Check sheet for the modelled part. Datum: model origin and axes. Units: mm. A direction names the side the tool comes from. Round coordinates to 2 decimals unless told otherwise and drop trailing zeros. Loops run counter-clockwise (first coordinate to the right, second up) from the corner with the lowest first, then second, coordinate; pieces in that order, holes last. Notation, with made-up numbers: (-13, 31) - (25, 31) arc R31 cw to (25, 61) - close; hole circle Ø10 at (11.25, 82.25). An arc over 180 degrees is marked (long way). Return JSON: item names as keys, results as strings.
from build123d import *

# Parameters (mm, degrees)
F0_W     = 228.6
F0_H     = 101.6
F0_W_2   = 39.424618
F0_H_2   = 25.4
F0_W_3   = 38.1
F1_DEPTH = 38.1
F2_DEPTH = 25.4


with BuildPart() as f1:
    # F0 (on Front) → F1 (new body)
    with BuildSketch(Plane.XZ):
        Rectangle(F0_W, F0_H)
        Polygon((-63.5, -38.1), (-101.6, -38.1), (-101.6, -12.7), (-101.6, 12.7), (-101.6, 38.1), (-62.175382, 38.1), (63.5, 38.1), (101.6, 38.1), (101.6, 12.7), (101.6, -12.7), (101.6, -38.1), (63.5, -38.1), align=None, mode=Mode.SUBTRACT)
        with Locations((-81.887691, 25.4)):
            Rectangle(F0_W_2, F0_H_2)
        Polygon((-63.5, -12.7), (-63.5, -38.1), (63.5, -38.1), (63.5, -12.7), (101.6, -12.7), (101.6, 12.7), (63.5, 12.7), (63.5, 38.1), (-62.175382, 38.1), (-62.175382, 12.7), (-101.6, 12.7), (-101.6, -12.7), align=None)
        with Locations((-23.794951, 0)):
            Rectangle(F0_W_3, F0_H_2, mode=Mode.SUBTRACT)
        with Locations((30.221954, 0)):
            Rectangle(F0_W_3, F0_H_2, mode=Mode.SUBTRACT)
        with Locations((-23.794951, 0)):
            Rectangle(F0_W_3, F0_H_2)
        with Locations((-82.55, -25.4)):
            Rectangle(F0_W_3, F0_H_2)
        with Locations((30.221954, 0)):
            Rectangle(F0_W_3, F0_H_2)
        with Locations((82.55, -25.4)):
            Rectangle(F0_W_3, F0_H_2)
        with Locations((82.55, 25.4)):
            Rectangle(F0_W_3, F0_H_2)
    extrude(amount=-F1_DEPTH)

    # F0 (on Front) → F2 (cut)
    with BuildSketch(Plane.XZ):
        with Locations((-81.887691, 25.4)):
            Rectangle(F0_W_2, F0_H_2)
        with Locations((-82.55, -25.4)):
            Rectangle(F0_W_3, F0_H_2)
        with Locations((-23.794951, 0)):
            Rectangle(F0_W_3, F0_H_2)
        with Locations((30.221954, 0)):
            Rectangle(F0_W_3, F0_H_2)
        with Locations((82.55, 25.4)):
            Rectangle(F0_W_3, F0_H_2)
        with Locations((82.55, -25.4)):
            Rectangle(F0_W_3, F0_H_2)
    extrude(amount=-F2_DEPTH, mode=Mode.SUBTRACT)


solid = f1.part
Q1. Tool access check on faces 1 (the face through (114.3, 19, -1)), 2 (the face through (30, 25.4, 0)). Record the directions out of +Z, -Z, +X, -X, +Y, -Y that give a thin tool (end or side, any length) a straight path to the whole face; none if there is none.
Answer key:
{"face 1": "+Z, -Z, +X, +Y, -Y", "face 2": "-Y"}
Q2. Depth check by flat-ended pin: P1, Ø7.5, axis at x = -26.5, z = 5, coming from the -Y side. Enter the tip coordinate at first touch or a pass-through.
Answer key:
{"P1": "stops at y = 25.4"}
Q3. Draft check along Z on faces 3 (the face through (-2, 19, -50.8)), 4 (the face through (30, 13, 12.7)), 5 (the face through (-24, 25.4, 0)), 6 (the face through (-2, 0, 1)). Enter one of: released by +Z, released by -Z, zero draft, split by the parting line, or undercut.
Answer key:
{"face 3": "released by -Z", "face 4": "undercut", "face 5": "undercut", "face 6": "zero draft"}
Q4. Sectioned sample at A-A (z = -25.5). Enter the section's corners in (x, y), plus the area to 3 significant figures.
Answer key:
{"outline": "(-114.3, 0) - (-101.6, 0) - (-101.6, 25.4) - (-63.5, 25.4) - (-63.5, 0) - (63.5, 0) - (63.5, 25.4) - (101.6, 25.4) - (101.6, 0) - (114.3, 0) - (114.3, 38.1) - (-114.3, 38.1) - close", "area": "6,770 mm²"}
Q5. Sectioned sample at C-C (x = -72). Enter the section's corners in (y, z), plus the area to 3 significant figures.
Answer key:
{"outline": "(0, -50.8) - (38.1, -50.8) - (38.1, 50.8) - (0, 50.8) - (0, 38.1) - (25.4, 38.1) - (25.4, 12.7) - (0, 12.7) - (0, -12.7) - (25.4, -12.7) - (25.4, -38.1) - (0, -38.1) - close", "area": "2,580 mm²"}
Q6. Sectioned sample at B-B (y = 8.5). Enter the section's corners in (x, z), plus the area to 3 significant figures.
Answer key:
{"outline": "(-114.3, -50.8) - (114.3, -50.8) - (114.3, 50.8) - (-114.3, 50.8) - close; hole (-101.6, -38.1) - (-63.5, -38.1) - (-63.5, -12.7) - (-101.6, -12.7) - close; hole (-101.6, 12.7) - (-62.18, 12.7) - (-62.18, 38.1) - (-101.6, 38.1) - close; hole (-42.84, -12.7) - (-4.74, -12.7) - (-4.74, 12.7) - (-42.84, 12.7) - close; hole (11.17, -12.7) - (49.27, -12.7) - (49.27, 12.7) - (11.17, 12.7) - close; hole (63.5, -38.1) - (101.6, -38.1) - (101.6, -12.7) - (63.5, -12.7) - close; hole (63.5, 12.7) - (101.6, 12.7) - (101.6, 38.1) - (63.5, 38.1) - close", "area": "17,400 mm²"}
Q7. Sectioned sample at D-D (x = -34.5). Enter the section's corners in (y, z), plus the area to 3 significant figures.
Answer key:
{"outline": "(0, -50.8) - (38.1, -50.8) - (38.1, 50.8) - (0, 50.8) - (0, 12.7) - (25.4, 12.7) - (25.4, -12.7) - (0, -12.7) - close", "area": "3,230 mm²"}
Q8. Scan lines: probe 1 along X at (y, z) = (2, 6.5); probe 2 along X at (y, z) = (6, -37.5); probe 3 along Z at (x, y) = (101.5, 14.5). Record each from-to range of solid material in increasing order. Write a range as [from, to].
Answer key:
{"probe 1": "x = [-114.3, -42.84], [-4.74, 11.17], [49.27, 114.3]", "probe 2": "x = [-114.3, -101.6], [-63.5, 63.5], [101.6, 114.3]", "probe 3": "z = [-50.8, -38.1], [-12.7, 12.7], [38.1, 50.8]"}
